The drawing under review shows one solid part. Ordinate dimensions are in mm from its lowest x, y, z. A direction names the side the tool comes from. Coordinates: 2 decimals unless noted, no trailing zeros. Order: outer loops, then holes, each group sorted by start corner. A loop starts at its lowest first (then second) coordinate and runs counter-clockwise, first axis right, second up. Notation, with made-up numbers: (3.25, 19.5) - (60.25, 19.5) arc R25 cw to (60.25, 50.5) - close; hole circle Ø10 at (-33.5, 89.5). An arc over 180 degrees is marked (long way). Answer in a Markdown table with one row per item.
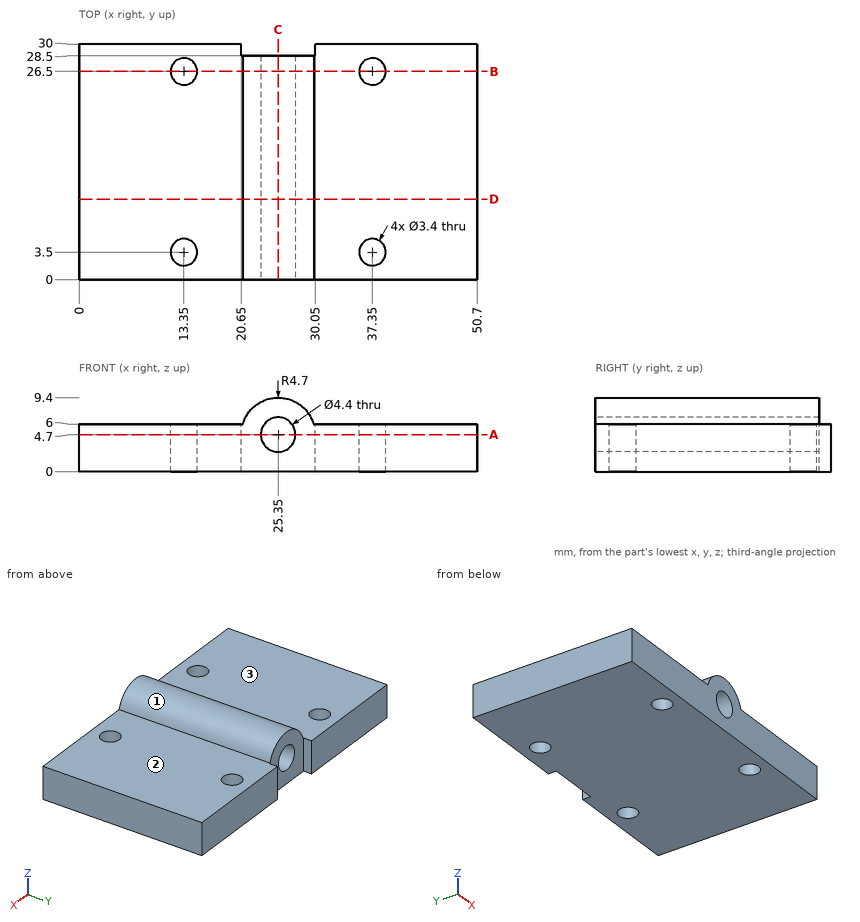
Item 1: Tool access review of the marked faces 1, 2 and 3: name each direction out of +Z, -Z, +X, -X, +Y, -Y from which nothing blocks a thin tool from reaching the whole face with its end or side.
Check values:
| item | result |
|---|---|
| face 1 | +Z, +Y, -Y |
| face 2 | +Z, +X, +Y, -Y |
| face 3 | +Z, -X, +Y, -Y |
Item 2: We need section C-C, the plane x = 25.35. Write out the cut boundary in (y, z), then the cut area to 4 significant figures.
Check values:
| item | result |
|---|---|
| outline | (0, 0) - (28.5, 0) - (28.5, 2.5) - (0, 2.5) - close; (0, 6.9) - (28.5, 6.9) - (28.5, 9.4) - (0, 9.4) - close |
| area | 142.5 mm^2 |
Item 3: To check wall thickness, follow line 1 (Y direction, x = 37.35, z = 4); line 2 (X direction, y = 11.75, z = 4.5); line 3 (X direction, y = 27.5, z = 5.75). State the ranges of each line that lie inside material, in increasing order. Write a range as from..to.
Check values:
| item | result |
|---|---|
| line 1 | 0..1.8, 5.2..24.8, 28.2..30 |
| line 2 | 0..23.16, 27.54..50.7 |
| line 3 | 0..11.98, 14.72..23.42, 27.28..35.98, 38.72..50.7 |
Item 4: Clearance check with flat-ended pins moving along their axes: pin 1 Ø10.5 at (x, y) = (39, 16) entering from +Z; pin 2 Ø4.5 at (x, z) = (25, 5.5) entering from +Y. State where each tip first meets the part, or that it passes through.
Check values:
| item | result |
|---|---|
| pin 1 | z = 6 |
| pin 2 | y = 28.5 |
Item 5: We need section B-B, the plane y = 26.5. Write out the cut boundary in (x, z), then the cut area to 3 significant figures.
Check values:
| item | result |
|---|---|
| outline | (0, 0) - (11.65, 0) - (11.65, 6) - (0, 6) - close; (15.05, 0) - (35.65, 0) - (35.65, 6) - (29.87, 6) arc R4.7 ccw to (20.83, 6) - (15.05, 6) - close; (39.05, 0) - (50.7, 0) - (50.7, 6) - (39.05, 6) - close; hole circle Ø4.4 at (25.35, 4.7) |
| area | 271 mm^2 |
Item 6: We need section A-A, the plane z = 4.7. Write out the cut boundary in (x, y).
Check values:
| item | result |
|---|---|
| outline | (0, 0) - (23.15, 0) - (23.15, 28.5) - (20.65, 28.5) - (20.65, 30) - (0, 30) - close; (27.55, 0) - (50.7, 0) - (50.7, 30) - (30.05, 30) - (30.05, 28.5) - (27.55, 28.5) - close; hole circle Ø3.4 at (13.35, 3.5); hole circle Ø3.4 at (13.35, 26.5); hole circle Ø3.4 at (37.35, 3.5); hole circle Ø3.4 at (37.35, 26.5) |
Item 7: We need section D-D, the plane y = 10.25. Write out the cut boundary in (x, z).
Check values:
| item | result |
|---|---|
| outline | (0, 0) - (50.7, 0) - (50.7, 6) - (29.87, 6) arc R4.7 ccw to (20.83, 6) - (0, 6) - close; hole circle Ø4.4 at (25.35, 4.7) |
